The listing builds one solid part. Answer for the finished solid, in the listing's coordinates (mm). Face numbers are marked on the shaded views. A direction names the side the tool comes from. Coordinates: 2 decimals unless noted, no trailing zeros. Order: outer loops, then holes, each group sorted by start corner. A loop starts at its lowest first (then second) coordinate and runs counter-clockwise, first axis right, second up. Notation, with made-up numbers: M 48,25 L 97,25 A14 ccw 97,37 Z; hole C 37.5,-33 d3. An arc over 180 degrees is marked long. One line per item, written item: value. Start each with the question number.
Q1. The part is cut by section A-A on z = 29. Give the vertices of the cut face in (x, y).
Q2. The part is cut by section D-D on z = 73. Give the vertices of the cut face in (x, y), then the cut area to 3 significant figures.
Q3. The part is cut by section C-C on y = 5.5. Give the vertices of the cut face in (x, z), then the cut area to 3 significant figures.
Q4. The part is cut by section B-B on x = -5. Give the vertices of the cut face in (y, z).
Q5. Each of these flat-tipped pins is pushed along its axis until it touches: pin 1 Ø1.8 at (y, z) = (-5, 63) entering from +X; pin 2 Ø1.8 at (x, z) = (-6, 73.5) entering from -Y; pin 3 Ø10 at (x, z) = (-3.5, 44.5) entering from -Y. Where does it stop, or does it pass through?
Q6. For the marked faces 1 and 2, determine the directions among +Z, -Z, +X, -X, +Y, -Y from which every point of the face is accessible in a straight line to the end or side of a thin tool.
Q7. Straight lines are drawn through the part: line 1 along X through (y, z) = (-6.5, 71.5); line 2 along Y through (x, z) = (-0.25, 40). For each, find the intervals that lie inside material, in ascending order. Write a range as [from, to].
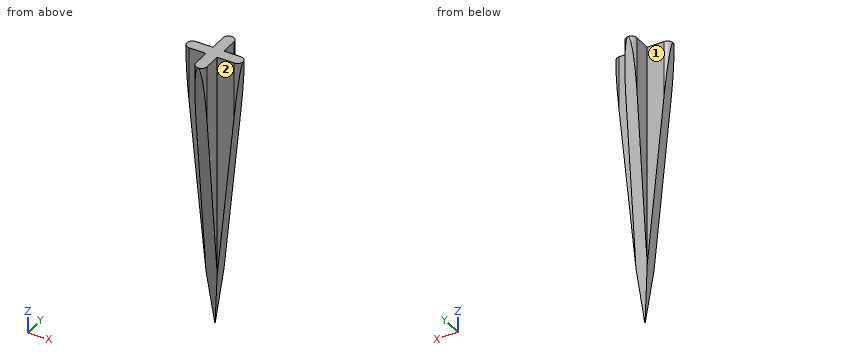
Autodesk Inventor part; units mm, degrees
ref_plane "YZ Plane" through (0, 0, 0) normal (1, 0, 0) x (0, 1, 0)
ref_plane "XZ Plane" through (0, 0, 0) normal (0, 1, 0) x (-1, 0, 0)
ref_plane "XY Plane" through (0, 0, 0) normal (0, 0, 1) x (1, 0, 0)
sketch "Sketch1" plane through (0, 0, 0) normal (0, 0, 1) x (1, 0, 0)
  line L0 (0, 0) -> (0, -10)
  line L1 (0, 0) -> (10, 0)
  line L2 (0, 0) -> (0, 10)
  line L3 (0, 0) -> (-10, 0)
  line L4 (-10, 0) -> (-10, -2)
  line L5 (-10, -2) -> (0, -2)
  line L6 (-10, 0) -> (-10, 2)
  line L7 (-10, 2) -> (0, 2)
  line L8 (0, 10) -> (-2, 10)
  line L9 (-2, 10) -> (-2, 0)
  line L10 (0, 10) -> (2, 10)
  line L11 (2, 10) -> (2, 0)
  line L12 (0, 2) -> (10, 2)
  line L13 (10, 2) -> (10, 0)
  line L14 (10, -2) -> (0, -2)
  line L15 (10, -2) -> (10, 0)
  line L16 (2, 0) -> (2, -10)
  line L17 (0, -10) -> (2, -10)
  line L18 (0, -10) -> (-2, -10)
  line L19 (-2, -10) -> (-2, 0)
  line L20 (-10, 0) -> (-8, 0)
  line L21 (-8, 0) -> (-8, -2)
  line L22 (-8, 0) -> (-8, 2)
  arc A0 (-8, 2) -> (-10, 0) centre (-8, 0) ccw
  arc A1 (-10, 0) -> (-8, -2) centre (-8, 0) ccw
  line L23 (0, -10) -> (0, -8)
  line L24 (0, -8) -> (2, -8)
  line L25 (0, -8) -> (-2, -8)
  arc A2 (-2, -8) -> (0, -10) centre (0, -8) ccw
  arc A3 (0, -10) -> (2, -8) centre (0, -8) ccw
  line L26 (10, 0) -> (8, 0)
  line L27 (8, 0) -> (8, 2)
  line L28 (8, 0) -> (8, -2)
  arc A4 (8, -2) -> (10, 0) centre (8, 0) ccw
  arc A5 (10, 0) -> (8, 2) centre (8, 0) ccw
  line L29 (0, 10) -> (0, 8)
  line L30 (0, 8) -> (2, 8)
  line L31 (0, 8) -> (-2, 8)
  arc A6 (0, 10) -> (-2, 8) centre (0, 8) ccw
  arc A7 (2, 8) -> (0, 10) centre (0, 8) ccw
  point P0 (-2, -2)
  point P1 (2, -2)
  point P2 (2, 2)
  point P3 (-2, 2)
  dimension "d0" = 10
  dimension "d1" = 10
  dimension "d2" = 10
  dimension "d3" = 10
  dimension "d4" = 2
  dimension "d5" = 2
  dimension "d6" = 2
  dimension "d7" = 2
  dimension "d8" = 2
  dimension "d9" = 2
  dimension "d10" = 2
  dimension "d11" = 2
  dimension "d12" = 2
  dimension "d13" = 2
  dimension "d14" = 2
  dimension "d15" = 2
  dimension "d16" = 2
  dimension "d17" = 2
  dimension "d18" = 2
extrude "Extrusion1" add sketch "Sketch1" along normal blind 100 contours L1 L16 L14 L0 | L2 L12 L11 L1 | L3 L9 L7 L2 | L0 L5 L19 L3 | L14 L16 L24 L0 | L0 L25 L19 L5 | L11 L12 L27 L1 | L1 L28 L14 L16 | L7 L9 L31 L2 | L2 L30 L11 L12 | L19 L5 L21 L3 | L3 L22 L7 L9 | L24 A3 L0 | L0 A2 L25 | L27 A5 L1 | L1 A4 L28 | L31 A6 L2 | L2 A7 L30 | L21 A1 L3 | L3 A0 L22
sketch "Sketch2" plane through (0, 0, 0) normal (0, 1, 0) x (-1, 0, 0)
  line L0 (2, 100) -> (-2, 100)
  line L1 (10, 0) -> (10, 100)
  line L2 (2, 100) -> (2, 0)
  line L3 (10, 100) -> (2, 100)
  line L4 (-2, 100) -> (-2, 0)
  line L5 (-8, 100) -> (-10, 100)
  line L6 (-10, 100) -> (-2, 100)
  line L7 (10, 0) -> (10, 100)
  line L8 (-2, 0) -> (-10, 0)
  line L9 (-10, 0) -> (-10, 100)
  line L10 (10, 0) -> (0, 0)
  line L11 (0, 0) -> (10, 100)
  line L12 (0, 0) -> (-10, 100)
  line L13 (-10, 0) -> (0, 0)
  line L14 (0, 0) -> (-10, 100)
extrude "Extrusion2" cut sketch "Sketch2" along normal mid plane 20 contours L11 L1 L10 L2 | L2 L10 L11 | L12 L13 L4 | L4 L8 L9 L12
sketch "Sketch3" plane through (0, 0, 0) normal (1, 0, 0) x (0, 1, 0)
  line L0 (0, 100) -> (-2, 100)
  line L1 (0, 0) -> (0, 100)
  line L2 (0, 100) -> (10, 100)
  line L3 (10, 0) -> (10, 100)
  line L4 (10, 100) -> (10, 0)
  line L5 (-10, 0) -> (10, 0)
  line L6 (0, 0) -> (10, 0)
  line L7 (10, 0) -> (0, 0)
  line L8 (10, 100) -> (0, 0)
  line L9 (0, 0) -> (-10, 0)
  line L10 (-10, 0) -> (-10, 100)
  line L11 (-10, 100) -> (0, 100)
  line L12 (-10, 100) -> (0, 0)
extrude "Extrusion3" cut sketch "Sketch3" along normal mid plane 20 contours L8 L3 L5 | L5 L10 L12
sketch "Sketch4" plane through (0, 0, 100) normal (0, 0, 1) x (1, 0, 0)
  line L0 (-8, -2) -> (-2, -2)
  line L1 (-2, -2) -> (-8, -2)
  line L2 (-2, -2) -> (-2, -7.923)
  line L3 (2, -8) -> (2, -2)
  line L4 (2, -2) -> (2, -8)
  arc A0 (8, -2) -> (10, 0) centre (8, 0) ccw
  line L5 (2, -2) -> (8, -2)
  line L6 (2, 2) -> (2, 8)
  line L7 (8, 2) -> (2, 2)
  line L8 (2, 2) -> (8, 2)
  line L9 (2, 2) -> (2, 8)
  line L10 (-2, 8) -> (-2, 2)
  line L11 (-2, 2) -> (-2, 8)
  arc A1 (-8, 2) -> (-10, 0) centre (-8, 0) ccw
  line L12 (-2, 2) -> (-8, 2)
  arc A2 (-8, 2) -> (-8, -2) centre (-8, 0) ccw
  arc A3 (-2, -8) -> (0, -10) centre (0, -8) ccw
  arc A4 (-2, -8) -> (2, -8) centre (0, -8) ccw
  arc A5 (8, -2) -> (8, 2) centre (8, 0) ccw
  arc A6 (2, 8) -> (-2, 8) centre (0, 8) ccw
properties part number "Prikker V1.1" material "ABS Plastic"
Output:
1. outline: M -2.9,-2 L -2,-2 L -2,-2.9 L 2,-2.9 L 2,-2 L 2.9,-2 L 2.9,2 L 2,2 L 2,2.9 L -2,2.9 L -2,2 L -2.9,2 Z
2. outline: M -7.3,-2 L -2,-2 L -2,-7.3 L 2,-7.3 L 2,-2 L 7.3,-2 L 7.3,2 L 2,2 L 2,7.3 L -2,7.3 L -2,2 L -7.3,2 Z
2. area: 101 mm^2
3. outline: M -2,55 L 2,55 L 2,100 L -2,100 Z
3. area: 180 mm^2
4. outline: M -2,50 L 2,50 L 2,100 L -2,100 Z
5. pin 1: stops at x = 2
5. pin 2: stops at y = -2
5. pin 3: stops at y = -4.93
6. face 1: +Z, -Z, -X, +Y
6. face 2: +Z, -Z, +X, -Y
7. line 1: x = [-2, 2]
7. line 2: y = [-4, 4]
